from build123d import *

# Parameters (mm, degrees)
F1_DEPTH      = 1.5875
F1_DEPTH_BACK = 1.5875


with BuildPart() as f1:
    # F0 (on Front) → F1 (new body, two sides)
    with BuildSketch(Plane.XZ) as f1_sk:
        with BuildLine():
            Line((68.744436, 6.35), (68.744436, 12.7))
            Line((68.744436, 12.7), (-64.605564, 12.7))
            ThreePointArc((-64.605564, 12.7), (-69.095692, 10.840128), (-70.955564, 6.35))
            Line((-70.955564, 6.35), (-66.193064, 6.35))
            ThreePointArc((-66.193064, 6.35), (-64.605564, 7.9375), (-63.018064, 6.35))
            Line((-63.018064, 6.35), (60.806936, 6.35))
            ThreePointArc((60.806936, 6.35), (62.394436, 7.9375), (63.981936, 6.35))
            Line((63.981936, 6.35), (68.744436, 6.35))
        make_face()
        with BuildLine():
            Line((68.744436, 0), (68.744436, 6.35))
            Line((68.744436, 6.35), (63.981936, 6.35))
            ThreePointArc((63.981936, 6.35), (62.394436, 4.7625), (60.806936, 6.35))
            Line((60.806936, 6.35), (-63.018064, 6.35))
            ThreePointArc((-63.018064, 6.35), (-64.605564, 4.7625), (-66.193064, 6.35))
            Line((-66.193064, 6.35), (-70.955564, 6.35))
            ThreePointArc((-70.955564, 6.35), (-69.095692, 1.859872), (-64.605564, 0))
            Line((-64.605564, 0), (68.744436, 0))
        make_face()
    extrude(amount=F1_DEPTH)
    extrude(f1_sk.sketch, amount=-F1_DEPTH_BACK)


solid = f1.part
CAD build for the part. Positions are in the model's coordinates, mm. Give positions to 0.01 mm unless a question says otherwise; leave off trailing zeros. Write each question's results on one line, items separated by ' | '.
1. Saw through at A-A on y = -0.3. Count the separate pieces of the cut face and the enclosed holes in it, and give its area (3 significant figures).
Calculated:
separate pieces: 1 | enclosed holes: 2 | area: 1,740 mm2
2. Probe L1, parallel to Z at x = 62, y = 1.05; L2, parallel to X at y = -0.6, z = 10.75; L3, parallel to X at y = -0.3, z = 3. List the from-to ranges inside material, lowest first. Write a range as from..to.
Calculated:
L1: z = 0..4.81, 7.89..12.7 | L2: x = -69.18..68.74 | L3: x = -70..68.74
3. Pull direction Z, two halves, no side cores. Call faces 1 (the face through (60.81, -0.02, 6.28)), 2 (the face through (-2, 1.588, 6)), 3 (the face through (1, 0, 0)): released by +Z, released by -Z, zero draft, split by the parting line, or undercut.
Calculated:
face 1: undercut | face 2: zero draft | face 3: released by -Z
